```python
from build123d import *

# Parameters (mm, degrees)
K_TOWNIK_STALOWY_35_X_35_X_5_1_DEPTH = 158
SZKIC3_R                             = 5
WYTNIJ_WYCI_GNI_CIE1_DEPTH           = 10


with BuildPart() as part:
    # Sketch1 → Kątownik stalowy 35 X 35 X 5(1) (new body)
    with BuildSketch(Plane.YX.offset(-79)):
        with BuildLine():
            Line((0, 0), (0, 35))
            ThreePointArc((0, 35), (3.535533906, 33.535533906), (5, 30))
            Line((5, 30), (5, 10))
            ThreePointArc((5, 10), (6.464466094, 6.464466094), (10, 5))
            Line((10, 5), (30, 5))
            ThreePointArc((30, 5), (33.535533906, 3.535533906), (35, 0))
            Line((35, 0), (0, 0))
        make_face()
    extrude(amount=K_TOWNIK_STALOWY_35_X_35_X_5_1_DEPTH)

    # Szkic3 → Wytnij-wyciągnięcie1 (cut)
    with BuildSketch(Plane.ZY):
        with Locations((44, 26.5)):
            Circle(SZKIC3_R)
    extrude(amount=-WYTNIJ_WYCI_GNI_CIE1_DEPTH, mode=Mode.SUBTRACT)


solid = part.part
```
CAD build for the part. Positions are in the model's coordinates, mm. A direction names the side the tool comes from. Round coordinates to 2 decimals unless told otherwise and drop trailing zeros. Loops run counter-clockwise (first coordinate to the right, second up) from the corner with the lowest first, then second, coordinate; pieces in that order, holes last. Notation, with made-up numbers: (32, -4.75) - (82, -4.75) arc R25 ccw to (82, 12.25) - close; hole circle Ø9 at (42.25, 0). An arc over 180 degrees is marked (long way). Return JSON: item names as keys, results as strings. Group by question number.
Q1. Tool access for faces 1 (the face through (0, 18, 1)), 2 (the face through (20, 5, 1)): list every direction of +Z, -Z, +X, -X, +Y, -Y with a clear straight run to the whole face (end or side of a thin tool).
Q2. Flat gauge pins, fed straight in: pin 1 Ø5 at (x, z) = (27.5, 43) entering from +Y; pin 2 Ø12 at (x, z) = (6, 48.5) entering from +Y; pin 3 Ø9 at (y, z) = (26.5, 44) entering from -X (3 decimals). Where does each tip first touch, or does it go through?
Q3. Band-saw the part on B-B on z = 44. Give the cut face in (x, y), plus the area to 3 significant figures.
Q4. Band-saw the part on C-C on y = 33. Give the cut face in (x, z).
Q5. Drill centre lines: line 1 along Z through (x, y) = (2.4, 26.5); line 2 along X through (y, z) = (19.5, 58.5). Where is each one in solid material? Low to high. Write a range as [from, to].
Q6. Band-saw the part on D-D on x = 8.5. Give the cut face in (y, z).
Q7. Band-saw the part on A-A on y = 26.5. Give the cut face in (x, z), plus the area to 3 significant figures.
Q8. Two-plate mould, pull along Y, no slides. Class faces 3 (the face through (2.5, 23.5, 40)), 4 (the face through (4.6, 9.8, 79)), 5 (the face through (34, 3, 1)), 6 (the face through (17, 0, 1)): +Y half, -Y half, draft (parallel to the pull), parting line (faces both ways), or undercut.
Solutions:
{
 "1": {"face 1": "+Z, -Z, -X, +Y, -Y", "face 2": "+Z, -Z, +X, +Y"},
 "2": {"pin 1": "stops at y = 5", "pin 2": "stops at y = 35", "pin 3": "passes through"},
 "3": {"outline": "(0, 0) - (35, 0) arc R5 ccw to (30, 5) - (10, 5) arc R5 cw to (5, 10) - (5, 21.5) - (0, 21.5) - close; (0, 31.5) - (4.77, 31.5) arc R5 ccw to (0, 35) - close", "area": "270 mm^2"},
 "4": {"outline": "(0, -79) - (4, -79) - (4, 79) - (0, 79) - close"},
 "5": {"line 1": "z = [-79, 39], [49, 79]", "line 2": "x = [0, 5]"},
 "6": {"outline": "(0, -79) - (5.23, -79) - (5.23, 79) - (0, 79) - close"},
 "7": {"outline": "(0, -79) - (5, -79) - (5, 39) - (0, 39) - close; (0, 49) - (5, 49) - (5, 79) - (0, 79) - close", "area": "740 mm^2"},
 "8": {"face 3": "undercut", "face 4": "draft", "face 5": "+Y half", "face 6": "-Y half"}
}
